```python
from build123d import *

# Parameters (mm, degrees)
SKETCH1_R           = 8.025
SKETCH1_R_2         = 2.45
BOSS_EXTRUDE1_DEPTH = 16
SKETCH3_W           = 7
SKETCH3_H           = 1.95


with BuildPart() as part:
    # Sketch1 → Boss-Extrude1 (new body)
    with BuildSketch(Plane(origin=(0, 0, 0), x_dir=(0, 0, -1), z_dir=(1, 0, 0))):
        Circle(SKETCH1_R)
        Circle(SKETCH1_R_2, mode=Mode.SUBTRACT)
    extrude(amount=BOSS_EXTRUDE1_DEPTH)

    # Sketch3 → Cut-Revolve1 (revolve, cut)
    with BuildSketch(Plane.XY, mode=Mode.PRIVATE) as cut_revolve1_sk:
        with Locations((11, 7.05)):
            Rectangle(SKETCH3_W, SKETCH3_H)
    revolve(cut_revolve1_sk.sketch.rotate(Axis((-1.784254148, 0, 0), (1, 0, 0)), 90), axis=Axis((-1.784254148, 0, 0), (1, 0, 0)), mode=Mode.SUBTRACT)


solid = part.part
```
Read the model definition and answer for the solid it produces. Units are mm, in the model's axes. A direction names the side the tool comes from. Coordinates: 2 decimals unless noted, no trailing zeros. Write each loop counter-clockwise with the first axis right and the second up, starting at its lowest first coordinate (ties: lowest second). Pieces come first, ordered by that corner, then holes. Notation, with made-up numbers: (66, 50.25) -> (89, 50.25) arc R15 ccw to (89, 74.25) -> close; hole circle Ø3 at (39.5, 76.5). An arc over 180 degrees is marked (long way). Write item = value, one per line.
(1) For a pull along X with two mould halves and no side action, classify faces 3 (the face through (0, 2, -2)), 4 (the face through (14.5, -2, 6)), 5 (the face through (3.7, -4.88, 6.37)) as +X half, -X half, draft (parallel to the pull), parting line (faces both ways), or undercut.
From the geometry:
face_3 = -X half
face_4 = undercut
face_5 = draft
(2) Straight lines are drawn through the part: L1, parallel to Y at x = 3.5, z = 0 (3 decimals); L2, parallel to X at y = 2.75, z = 5.5; L3, parallel to Y at x = 13.25, z = 2. For each, find the intervals that lie inside material, in ascending order. Write a range as from..to.
From the geometry:
L1 = -8.025..-2.45, 2.45..8.025
L2 = 0..7.5, 14.5..16
L3 = -5.74..-1.42, 1.42..5.74
(3) Section D-D on z = 4.5 is taken. Write down the section's boundary in (x, y).
From the geometry:
outline = (0, -6.64) -> (7.5, -6.64) -> (7.5, -4.08) -> (14.5, -4.08) -> (14.5, -6.64) -> (16, -6.64) -> (16, 6.64) -> (14.5, 6.64) -> (14.5, 4.08) -> (7.5, 4.08) -> (7.5, 6.64) -> (0, 6.64) -> close
(4) Which of the six approach directions +Z, -Z, +X, -X, +Y, -Y give full straight-line access (tool end or side, diameter ignored) to faces 1 (the face through (11.049, -1.825, 5.794)), 2 (the face through (7.9, -2.4, 0.5))?
From the geometry:
face_1 = none
face_2 = +X, -X
(5) Given pin 1 Ø6 at (x, z) = (4.5, -1.5) entering from -Y (3 decimals); pin 2 Ø1 at (x, z) = (4, 2) entering from +Y; pin 3 Ø3 at (x, y) = (7, -2) entering from -Z, each flat-ended and moving along its own axis, determine where each tip first touches the part or whether it passes through.
From the geometry:
pin_1 = -8.025
pin_2 = 7.88
pin_3 = -8.01
(6) Section C-C on x = 12 is taken. Write down the section's boundary in (y, z) (3 decimals), plus the area to 3 significant figures.
From the geometry:
outline = circle Ø12.15 at (0, 0); hole circle Ø4.9 at (0, 0)
area = 97.1 mm2
(7) Section A-A on z = 0 is taken. Write down the section's boundary in (x, y) (3 decimals).
From the geometry:
outline = (0, -8.025) -> (7.5, -8.025) -> (7.5, -6.075) -> (14.5, -6.075) -> (14.5, -8.025) -> (16, -8.025) -> (16, -2.45) -> (0, -2.45) -> close; (0, 2.45) -> (16, 2.45) -> (16, 8.025) -> (14.5, 8.025) -> (14.5, 6.075) -> (7.5, 6.075) -> (7.5, 8.025) -> (0, 8.025) -> close
